The listing builds one solid part. Answer for the finished solid, in the listing's coordinates (mm). Face numbers are marked on the shaded views. A direction names the side the tool comes from. Round coordinates to 2 decimals unless told otherwise and drop trailing zeros. Loops run counter-clockwise (first coordinate to the right, second up) from the corner with the lowest first, then second, coordinate; pieces in that order, holes last. Notation, with made-up numbers: (-28.75, -5) -> (-3.75, -5) arc R32 ccw to (-3.75, 22) -> close; hole circle Ø7 at (79, 83). An arc over 180 degrees is marked (long way). Write each question's results on one line, items separated by ' | '. Start each with the question number.
Autodesk Inventor part; units mm, degrees
ref_plane "YZ Plane" through (0, 0, 0) normal (1, 0, 0) x (0, 1, 0)
ref_plane "XZ Plane" through (0, 0, 0) normal (0, 1, 0) x (-1, 0, 0)
ref_plane "XY Plane" through (0, 0, 0) normal (0, 0, 1) x (1, 0, 0)
sketch "Sketch1" plane through (0, 0, 0) normal (0, 0, 1) x (1, 0, 0)
  line L0 (27, 38.5) -> (-27, 38.5)
  line L1 (-27, 38.5) -> (-27, -38.5)
  line L2 (-27, -38.5) -> (27, -38.5)
  line L3 (27, -38.5) -> (27, 38.5)
  line L4 (27, 38.5) -> (-27, -38.5) construction
  line L5 (-27, 38.5) -> (27, -38.5) construction
  line L6 (-18, 29.5) -> (18, 29.5)
  line L7 (18, 29.5) -> (18, -29.5)
  line L8 (18, -29.5) -> (-18, -29.5)
  line L9 (-18, -29.5) -> (-18, 29.5)
  line L10 (0, 57.4351) -> (0, -57.4351)
  point P0 (0, 0)
  point P1 (0, 0)
  dimension "d0" = 77
  dimension "d1" = 54
  dimension "d2" = 59
  dimension "d3" = 36
  dimension "d4" = 18
  dimension "d5" = 29.5
extrude "Extrusion1" add sketch "Sketch1" along normal blind 18 contours L3 L2 L10 L8 L7 L6 L0 | L10 L6 L9 L8 L2 L1 L0
sketch "Sketch2" plane through (0, 0, 18) normal (0, 0, 1) x (1, 0, 0)
  line L0 (27, -38.5) -> (27, 38.5)
  line L1 (27, 38.5) -> (-27, 38.5)
  line L2 (-27, 38.5) -> (-27, -38.5)
  line L3 (-27, -38.5) -> (27, -38.5)
  line L4 (18, -29.5) -> (-18, -29.5)
  line L5 (-18, -29.5) -> (-18, 29.5)
  line L6 (-18, 29.5) -> (18, 29.5)
  line L7 (18, 29.5) -> (18, -29.5)
  line L8 (-27, 0) -> (26, 0)
  line L9 (0, 38.5) -> (0, -38.5)
  point P0 (0, 0)
  point P1 (-9.5, 34)
  point P2 (9.5, 34)
  point P3 (22.5, 34)
  point P4 (-22.5, 34)
  point P5 (-22.5, 21)
  point P6 (-22.5, 7)
  point P7 (-22.5, -7)
  point P8 (-22.5, -21)
  point P9 (-22.5, -34)
  point P10 (-9.5, -34)
  point P11 (9.5, -34)
  point P12 (22.5, -34)
  point P13 (-0.5, 0)
  point P14 (22.5, 21)
  point P15 (22.5, 7)
  point P16 (22.5, -7)
  point P17 (22.5, -21)
  dimension "d11" = 4.5
  dimension "d14" = 19
  dimension "d15" = 4.5
  dimension "d16" = 13
  dimension "d17" = 4.5
  dimension "d18" = 4.5
  dimension "d19" = 4.5
  dimension "d20" = 13
  dimension "d21" = 4.5
  dimension "d22" = 13
  dimension "d23" = 14
  dimension "d24" = 4.5
  dimension "d25" = 14
  dimension "d26" = 4.5
  dimension "d27" = 4.5
  dimension "d28" = 14
  dimension "d29" = 13
  dimension "d30" = 4.5
hole "Hole1" at (-9.5, 34, 18) at (9.5, 34, 18) at (22.5, 34, 18) at (-22.5, 34, 18) at (-22.5, 21, 18) at (-22.5, 7, 18) at (-22.5, -7, 18) at (-22.5, -21, 18) at (-22.5, -34, 18) at (-9.5, -34, 18) at (9.5, -34, 18) at (22.5, -34, 18) at (22.5, 21, 18) at (22.5, 7, 18) at (22.5, -7, 18) at (22.5, -21, 18) direction (0, 0, -1) diameter 4 end through all
sketch "Sketch3" plane through (-27, -38.5, 0) normal (0, -1, 0) x (1, 0, 0)
  line L0 (27, 0) -> (27, 18) construction
  line L1 (0, 18) -> (54, 18)
  line L2 (0, 0) -> (0, 18)
  line L3 (0, 9) -> (54, 9) construction
  line L4 (54, 0) -> (54, 18)
  point P0 (27, 9)
hole "Hole2" at (0, -38.5, 9) direction (0, 1, 0) diameter 6.647 depth 22.2
sketch "Sketch4" plane through (-27, 38.5, 0) normal (0, 1, 0) x (1, 0, 0)
  line L0 (27, 0) -> (27, -18) construction
  line L1 (0, -18) -> (54, -18)
  line L2 (54, 0) -> (54, -18)
  line L3 (54, -9) -> (0, -9) construction
  line L4 (0, 0) -> (0, -18)
  circle A0 centre (27, -9) radius 8
  dimension "d45" = 16
extrude "Extrusion2" add sketch "Sketch4" along normal blind 11
sketch "Sketch5" plane through (0, 49.5, 9) normal (0, 1, 0) x (1, 0, 0)
  circle A0 centre (0, 0) radius 3.3235
  circle A1 centre (0, 0) radius 8
  point P0 (0, 9)
hole "Hole3" at (0, 49.5, 9) direction (0, -1, 0) diameter 8.376 depth 27.3
sketch "Sketch6" plane through (27, -38.5, 0) normal (1, 0, 0) x (0, 0, -1)
  line L0 (0, 0) -> (0, 77)
  line L1 (0, 0) -> (0, 77)
  line L2 (0, 77) -> (-18, 77)
  line L3 (-18, 0) -> (-18, 77)
  line L4 (0, 0) -> (-18, 0)
  line L5 (0, 29.5) -> (-18, 29.5)
  line L6 (0, 19.5) -> (-18, 19.5)
  line L7 (0, 9) -> (-18, 9)
  line L8 (-9, 0) -> (-9, 77) construction
  point P0 (0, 38.5)
  point P1 (-9, 24)
hole "Hole4" at (27, -14.5, 9) direction (-1, 0, 0) diameter 6.647 depth 22.2
properties part number "HUDSON-1-32"
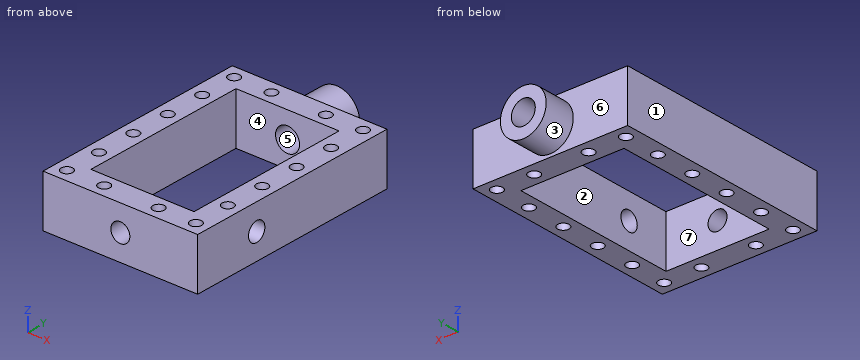
Item 1: For the marked faces 1, 2 and 3, determine the directions among +Z, -Z, +X, -X, +Y, -Y from which every point of the face is accessible in a straight line to the end or side of a thin tool.
Item 2: The part is cut by section C-C, the plane x = 9.5. Give the vertices of the cut face in (y, z).
Item 3: This flat-tipped pin is pushed along its axis until it touches: pin 1 Ø10 at (x, z) = (-16.5, 6.5) entering from +Y. Where does it stop, or does it pass through?
Item 4: The part is cut by section B-B, the plane y = -14.5. Give the vertices of the cut face in (x, z).
Item 5: Straight lines are drawn through the part: L1, parallel to X at y = 21, z = 10.5; L2, parallel to Y at x = 9.5, z = 11; L3, parallel to X at y = 27.5, z = 7.5. For each, find the intervals that lie inside material, in ascending order. Write a range as [from, to].
Item 6: Determine the mould class of the marked faces 4, 5, 6 and 7 for opening direction Y: +Y half, -Y half, draft (parallel to the pull), parting line (faces both ways), or undercut.
Item 7: The part is cut by section D-D, the plane y = -34. Give the vertices of the cut face in (x, z), plus the area to 3 significant figures.
Item 8: The part is cut by section A-A, the plane x = 22.5. Give the number of separate pieces and of enclosed holes in the cut face, plus the area to 3 significant figures.
Report:
1) face 1: +Z, -Z, -X, +Y, -Y | face 2: +Z, -Z | face 3: +Y
2) outline: (-38.5, 0) -> (-36, 0) -> (-36, 18) -> (-38.5, 18) -> close; (-32, 0) -> (-29.5, 0) -> (-29.5, 18) -> (-32, 18) -> close; (29.5, 0) -> (32, 0) -> (32, 18) -> (29.5, 18) -> close; (36, 0) -> (38.5, 0) -> (38.5, 18) -> (36, 18) -> close
3) pin 1: stops at y = 38.5
4) outline: (-27, 0) -> (-18, 0) -> (-18, 18) -> (-27, 18) -> close; (18, 0) -> (27, 0) -> (27, 5.68) -> (18, 5.68) -> close; (18, 12.32) -> (27, 12.32) -> (27, 18) -> (18, 18) -> close
5) L1: x = [-27, -24.5], [-20.5, -18], [18, 20.5], [24.5, 27] | L2: y = [-38.5, -36], [-32, -29.5], [29.5, 32], [36, 38.5] | L3: x = [-27, -18], [18, 27]
6) face 4: undercut | face 5: draft | face 6: +Y half | face 7: undercut
7) outline: (-27, 0) -> (-24.5, 0) -> (-24.5, 18) -> (-27, 18) -> close; (-20.5, 0) -> (-11.5, 0) -> (-11.5, 18) -> (-20.5, 18) -> close; (-7.5, 0) -> (7.5, 0) -> (7.5, 18) -> (-7.5, 18) -> close; (11.5, 0) -> (20.5, 0) -> (20.5, 18) -> (11.5, 18) -> close; (24.5, 0) -> (27, 0) -> (27, 18) -> (24.5, 18) -> close; hole circle Ø6.65 at (0, 9) | area: 649 mm2
8) separate pieces: 7 | enclosed holes: 1 | area: 919 mm2
